```python
from build123d import *

# Parameters (mm, degrees)
F1_DEPTH = 9.5
F3_DEPTH = 25
F4_R     = 2.5
F5_DEPTH = 7
F6_DEPTH = 25


with BuildPart() as f1:
    # F0 (on Front) → F1 (new body, symmetric)
    with BuildSketch(Plane.XZ):
        Polygon((0, 17), (0, 0), (13, 5), (13, 17), align=None)
    extrude(amount=F1_DEPTH, both=True)

    # F2 (on face) → F3 (cut)
    with BuildSketch(Plane.XY.offset(17)):
        Polygon((13, 9.5), (0, 9.5), (13, 4.5), align=None)
        Polygon((13, -9.5), (13, -4.5), (0, -9.5), align=None)
    extrude(amount=-F3_DEPTH, mode=Mode.SUBTRACT)

    # F4 (on Top) → F5 (cut)
    with BuildSketch(Plane.XY):
        with BuildLine():
            ThreePointArc((12, 1.5), (10.828427, 4.328427), (8, 5.5))
            Line((8, 5.5), (5, 5.5))
            ThreePointArc((5, 5.5), (2.171573, 4.328427), (1, 1.5))
            Line((1, 1.5), (1, -1.5))
            ThreePointArc((1, -1.5), (2.171573, -4.328427), (5, -5.5))
            Line((5, -5.5), (8, -5.5))
            ThreePointArc((8, -5.5), (10.828427, -4.328427), (12, -1.5))
            Line((12, -1.5), (12, 1.5))
        make_face()
        with Locations((6.5, 0)):
            Circle(F4_R, mode=Mode.SUBTRACT)
    extrude(amount=F5_DEPTH, mode=Mode.SUBTRACT)

    # F4 (on Top) → F6 (cut)
    with BuildSketch(Plane.XY):
        with Locations((6.5, 0)):
            Circle(F4_R)
    extrude(amount=F6_DEPTH, mode=Mode.SUBTRACT)


solid = f1.part
```
Could you check a few things on this model? Use its own coordinates, in mm. A direction names the side the tool comes from. Give positions to 0.01 mm unless a question says otherwise; leave off trailing zeros. Loops run counter-clockwise (first coordinate to the right, second up) from the corner with the lowest first, then second, coordinate; pieces in that order, holes last. Notation, with made-up numbers: (-39.5, 54) - (-35.5, 54) arc R32 ccw to (-35.5, 87) - close; hole circle Ø5 at (71.25, -21.5). An arc over 180 degrees is marked (long way). Use one line per item in the form item = value.
1. I want a section at A-A (x = 6.5). Please give me the cut outline in (y, z).
Response values:
outline = (-7, 2.5) - (-5.5, 2.5) - (-5.5, 7) - (-2.5, 7) - (-2.5, 17) - (-7, 17) - close; (2.5, 7) - (5.5, 7) - (5.5, 2.5) - (7, 2.5) - (7, 17) - (2.5, 17) - close
2. I'm going to push flat-ended pins straight in: pin 1 Ø1 at (x, z) = (4, 4) entering from -Y; pin 2 Ø5 at (x, z) = (10, 2.5) entering from +Y; pin 3 Ø1.5 at (x, z) = (6, 4) entering from -Y. Where does each tip first touch, or does it pass through?
Response values:
pin_1 = -8.15
pin_2 = 6.6
pin_3 = -7.48
3. I want a section at C-C (y = 2). Please give me the cut outline in (x, z), and give its area (3 significant figures).
Response values:
outline = (0, 0) - (1.03, 0.4) - (1.03, 7) - (5, 7) - (5, 17) - (0, 17) - close; (8, 7) - (11.97, 7) - (11.97, 4.6) - (13, 5) - (13, 17) - (8, 17) - close
area = 109 mm²
4. I want a section at D-D (x = 10.25). Please give me the cut outline in (y, z).
Response values:
outline = (-5.56, 3.94) - (-4.81, 3.94) - (-4.81, 7) - (4.81, 7) - (4.81, 3.94) - (5.56, 3.94) - (5.56, 17) - (-5.56, 17) - close
5. Thinking about a two-plate mould opening in X: for faces 3 (the face through (6.591, -6.965, 10.508)), 4 (the face through (10.859, 4.297, 5.447)), 5 (the face through (3.7, -0.1, 17)), which applies, released by +X, released by -X, zero draft, split by the parting line, or undercut?
Response values:
face_3 = released by +X
face_4 = undercut
face_5 = zero draft
6. I want a section at B-B (z = 6.5). Please give me the cut outline in (x, y).
Response values:
outline = (0, -9.5) - (13, -4.5) - (13, 4.5) - (0, 9.5) - close; hole (1, -1.5) arc R4 ccw to (5, -5.5) - (8, -5.5) arc R4 ccw to (12, -1.5) - (12, 1.5) arc R4 ccw to (8, 5.5) - (5, 5.5) arc R4 ccw to (1, 1.5) - close
7. On a 3-axis mill with a long thin cutter (end or side, diameter ignored), from which of +Z, -Z, +X, -X, +Y, -Y can I reach the whole of each face in a straight line? I mean faces 1 (the face through (13, 0, 11)), 2 (the face through (2.203, 4.359, 3.646)). Say none if no direction works.
Response values:
face_1 = +Z, -Z, +X, +Y, -Y
face_2 = -Z
8. I need wall thicknesses on probe 1 along X at (y, z) = (0, 11.75); probe 2 along Z at (x, y) = (4, 5); probe 3 along Y at (x, z) = (6.5, 10). Which ranges of each line are inside material? Lowest first, please.
Response values:
probe_1 = 0 to 4, 9 to 13
probe_2 = 7 to 17
probe_3 = -7 to -2.5, 2.5 to 7
